Geometry check sheet. Reference: the model listing, model coordinates, mm. Face numbers are marked on the shaded views. Coordinates: 2 decimals unless noted, no trailing zeros. Loops run counter-clockwise (first coordinate to the right, second up) from the corner with the lowest first, then second, coordinate; pieces in that order, holes last.
from build123d import *

# Parameters (mm, degrees)
F0_R     = 13.5255
F1_DEPTH = 49.911
F2_R     = 12.7635
F3_DEPTH = 49.149
F4_R     = 2.54
F4_R_2   = 1.5875
F5_DEPTH = 5.842
F6_R     = 1.5875
F7_DEPTH = 49.912


with BuildPart() as f1:
    # F0 (on Top) → F1 (new body)
    with BuildSketch(Plane.XY):
        Circle(F0_R)
    extrude(amount=-F1_DEPTH)

    # F2 (on face) → F3 (cut)
    with BuildSketch(Plane.XY):
        Circle(F2_R)
    extrude(amount=-F3_DEPTH, mode=Mode.SUBTRACT)

    # F4 (on face) → F5 (join)
    with BuildSketch(Plane(origin=(0, 0, -49.911), x_dir=(1, 0, 0), z_dir=(0, 0, -1))):
        Circle(F4_R)
        Circle(F4_R_2, mode=Mode.SUBTRACT)
    extrude(amount=-F5_DEPTH)

    # F6 (on face) → F7 (cut, through all)
    with BuildSketch(Plane(origin=(0, 0, -49.911), x_dir=(1, 0, 0), z_dir=(0, 0, -1))):
        Circle(F6_R)
    extrude(amount=-F7_DEPTH, mode=Mode.SUBTRACT)


solid = f1.part
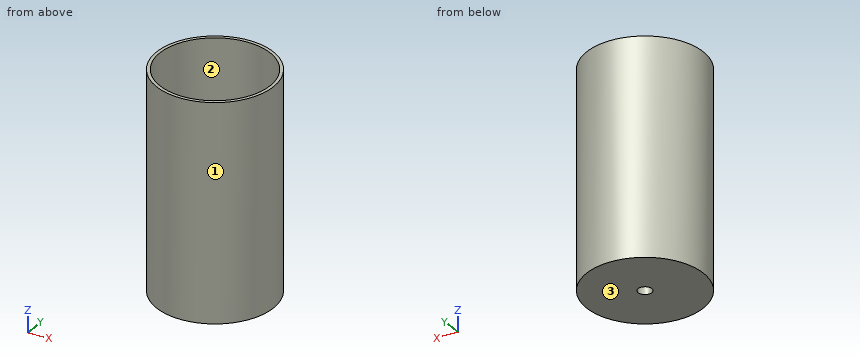
(1) Gauge pin test, flat ends, axial feed: pin 1 Ø1.5 at (x, y) = (6, 7) entering from +Z; pin 2 Ø1 at (y, z) = (-10.5, -20) entering from +X; pin 3 Ø5.5 at (x, y) = (-0.5, 0) entering from +Z. Record the tip position at first contact, or that the pin passes through.
Findings:
pin 1: stops at z = -49.15
pin 2: stops at x = 9.11
pin 3: stops at z = -44.07
(2) Draft check along X on the marked faces 1, 2 and 3. Enter one of: +X half, -X half, draft (parallel to the pull), parting line (faces both ways), or undercut.
Findings:
face 1: parting line
face 2: undercut
face 3: draft
(3) Sectioned sample at C-C on z = -45. Record the cut outline in (x, y) (1 decimal).
Findings:
outline: circle Ø27.1 at (0, 0); circle Ø5.1 at (0, 0); hole circle Ø25.5 at (0, 0); hole circle Ø3.2 at (0, 0)
(4) Sectioned sample at A-A on y = 0. Record the cut outline in (x, z), and give its area (3 significant figures).
Findings:
outline: (-13.53, -49.91) - (-1.59, -49.91) - (-1.59, -44.07) - (-2.54, -44.07) - (-2.54, -49.15) - (-12.76, -49.15) - (-12.76, 0) - (-13.53, 0) - close; (1.59, -49.91) - (13.53, -49.91) - (13.53, 0) - (12.76, 0) - (12.76, -49.15) - (2.54, -49.15) - (2.54, -44.07) - (1.59, -44.07) - close
area: 103 mm2
(5) Scan lines: L1, parallel to Y at x = 0, z = -45.95; L2, parallel to Y at x = 0, z = -28.5; L3, parallel to X at y = 0.5, z = -5.5. Record each from-to range of solid material in increasing order.
Findings:
L1: y = -13.53 to -12.76, -2.54 to -1.59, 1.59 to 2.54, 12.76 to 13.53
L2: y = -13.53 to -12.76, 12.76 to 13.53
L3: x = -13.52 to -12.75, 12.75 to 13.52
(6) Sectioned sample at D-D on x = 6.5. Record the cut outline in (y, z), and give its area (3 significant figures).
Findings:
outline: (-11.86, -49.91) - (11.86, -49.91) - (11.86, 0) - (10.98, 0) - (10.98, -49.15) - (-10.98, -49.15) - (-10.98, 0) - (-11.86, 0) - close
area: 104 mm2
